Geometry: final body of the model. Coordinates: model frame, mm. A direction names the side the tool comes from. Give positions to 0.01 mm unless a question says otherwise; leave off trailing zeros. Write each loop counter-clockwise with the first axis right and the second up, starting at its lowest first coordinate (ties: lowest second). Pieces come first, ordered by that corner, then holes.
Q1. Pin query (flat end, axial travel): pin 1 (2 mm diameter, centred on x = -70.79, z = 29.92, fed in from +Y); pin 2 (12 mm diameter, centred on x = 68.5, y = -27, fed in from +Z); pin 3 (19 mm diameter, centred on x = -37.85, z = 12.07, fed in from +Y); pin 4 (2.5 mm diameter, centred on x = 21, y = 2, fed in from -Z). Return the tip coordinate at first contact, or that it passes through.
Q2. Reachability of faces 4 (the face through (-98.077, -11, 5)), 5 (the face through (-36.045, 1.014, 17.789)) from +Z, -Z, +X, -X, +Y, -Y: full face, straight path, thin tool, end or side. Return the list, or none.
Q3. Line query: L1, parallel to Z at x = -5, y = -8.5; L2, parallel to X at y = -10, z = -15; L3, parallel to X at y = -15, z = -20. Output: solid intervals per line, ascending.
Q4. Draft query along Z for faces 1 (the face through (-98.081, -0.105, 4.671)), 2 (the face through (58.796, 1.014, 18.266)), 3 (the face through (-1, -10, 68.577)). Return one class per face: pulls with the +Z half, pulls with the -Z half, needs draft (parallel to the pull), parting line crosses it, or undercut.
Q5. Cut plane C-C on x = -2. Return the cut outline in (y, z), plus the area to 3 significant figures.
Q6. Cut plane B-B on y = -26. Return the cut outline in (x, z).
Q7. Cut plane A-A on y = -11.5. Return the cut outline in (x, z).
```python
from build123d import *

# Parameters (mm, degrees)
SKETCH1_W           = 160
SKETCH1_H           = 117
BOSS_EXTRUDE1_DEPTH = 2
SKETCH3_R           = 6
CUT_EXTRUDE1_DEPTH  = 100.127443223
SKETCH4_R           = 6
CUT_EXTRUDE3_DEPTH  = 100.127443223
SKETCH5_R           = 6
CUT_EXTRUDE4_DEPTH  = 100.127443223
SKETCH6_W           = 76.000007526
SKETCH6_H           = 46.999987397
SKETCH6_W_2         = 72.000007526
SKETCH6_H_2         = 42.999987397
CUT_EXTRUDE5_DEPTH  = 10
SKETCH7_R           = 4
SKETCH7_R_2         = 1.25
BOSS_EXTRUDE2_DEPTH = 7.81
SKETCH8_W           = 78.000007526
SKETCH8_H           = 48.999987397
SKETCH8_W_2         = 76.000007526
SKETCH8_H_2         = 46.999987397
BOSS_EXTRUDE3_DEPTH = 5.19
SKETCH9_W           = 76.000007526
SKETCH9_H           = 46.999987397
BOSS_EXTRUDE4_DEPTH = 2
DRAFT2_ANGLE        = 35
SKETCH12_W          = 160
SKETCH12_H          = 14.938358446
SKETCH12_W_2        = 31.199462864
SKETCH12_H_2        = 9.099678356
SKETCH12_W_3        = 31.607152295
SKETCH12_H_3        = 7.36210802
CUT_EXTRUDE7_DEPTH  = 10
SKETCH13_R          = 6
CUT_EXTRUDE8_DEPTH  = 10
SKETCH14_W          = 120
SKETCH14_H          = 2
SKETCH14_W_2        = 2
SKETCH14_H_2        = 47
SKETCH14_H_3        = 27
SKETCH14_H_4        = 20
BOSS_EXTRUDE5_DEPTH = 8
SKETCH15_R          = 5
SKETCH15_R_2        = 4
BOSS_EXTRUDE6_DEPTH = 33.22
CHAMFER1_SIZE       = 5
SKETCH16_R          = 1.25
CUT_EXTRUDE9_DEPTH  = 10


with BuildPart() as part:
    # Sketch1 → Boss-Extrude1 (new body)
    with BuildSketch(Plane(origin=(0, 0, 0), x_dir=(1, 0, 0), z_dir=(0, 1, 0))):
        Rectangle(SKETCH1_W, SKETCH1_H)
    extrude(amount=BOSS_EXTRUDE1_DEPTH)

    # Sketch3 → Cut-Extrude1 (cut, through all)
    with BuildSketch(Plane(origin=(0, 2, 0), x_dir=(1, 0, 0), z_dir=(0, 1, 0))):
        with Locations(Location((72.15303621, -2.066282122, 0), (0, 0, 270))):
            Circle(SKETCH3_R)
    extrude(amount=-CUT_EXTRUDE1_DEPTH, mode=Mode.SUBTRACT)

    # Sketch4 → Cut-Extrude3 (cut, through all)
    with BuildSketch(Plane(origin=(0, 2, 0), x_dir=(1, 0, 0), z_dir=(0, 1, 0))):
        with Locations(Location((23.553035896, -50.866150132, 0), (0, 0, 270))):
            Circle(SKETCH4_R)
    extrude(amount=-CUT_EXTRUDE3_DEPTH, mode=Mode.SUBTRACT)

    # Sketch5 → Cut-Extrude4 (cut, through all)
    with BuildSketch(Plane(origin=(0, 2, 0), x_dir=(1, 0, 0), z_dir=(0, 1, 0))):
        with Locations(Location((64.653036213, -19.566282124, 0), (0, 0, 270))):
            Circle(SKETCH5_R)
        with Locations(Location((-37.846967603, -12.066282143, 0), (0, 0, 270))):
            Circle(SKETCH5_R)
        with Locations(Location((1.053035896, -50.866150137, 0), (0, 0, 270))):
            Circle(SKETCH5_R)
        with Locations(Location((-53.91492316, 3.900994062, 0), (0, 0, 270))):
            Circle(SKETCH5_R)
        with Locations(Location((-70.34696951, -12.066282149, 0), (0, 0, 270))):
            Circle(SKETCH5_R)
        with Locations(Location((-54.14683932, -28.466289977, 0), (0, 0, 270))):
            Circle(SKETCH5_R)
    extrude(amount=-CUT_EXTRUDE4_DEPTH, mode=Mode.SUBTRACT)

    # Sketch6 → Cut-Extrude5 (cut)
    with BuildSketch(Plane(origin=(0, 2, 0), x_dir=(1, 0, 0), z_dir=(0, 1, 0))):
        with Locations((11.764130909, -9.702217308)):
            Rectangle(SKETCH6_W, SKETCH6_H)
        with Locations((11.764130909, -9.702217308)):
            Rectangle(SKETCH6_W_2, SKETCH6_H_2, mode=Mode.SUBTRACT)
    extrude(amount=-CUT_EXTRUDE5_DEPTH, mode=Mode.SUBTRACT)


with BuildPart() as cut_extrude5_kept_piece:
    # of the separate pieces the step leaves, the one the design keeps (cut_extrude5_pieces_kept)
    add(part.part.solids().sort_by_distance((80, 0, 58.5))[0])

    # Sketch7 → Boss-Extrude2 (add)
    # profile 1 of 5: a face of its own
    with BuildSketch(Plane.XZ):
        with Locations(Location((66.701777656, -9.076203809, 0), (0, 0, 90))):
            Circle(SKETCH7_R)
        with Locations(Location((66.701777656, -9.076203809, 0), (0, 0, 270))):
            Circle(SKETCH7_R_2, mode=Mode.SUBTRACT)
    # profile 2 of 5: a face of its own
    with BuildSketch(Plane.XZ):
        with Locations(Location((63.702108967, 46.190679909, 0), (0, 0, 90))):
            Circle(SKETCH7_R)
        with Locations(Location((63.702108967, 46.190679909, 0), (0, 0, 270))):
            Circle(SKETCH7_R_2, mode=Mode.SUBTRACT)
    # profile 3 of 5: a face of its own
    with BuildSketch(Plane.XZ):
        with Locations(Location((-31.54560253, 48.927228564, 0), (0, 0, 90))):
            Circle(SKETCH7_R)
        with Locations(Location((-31.54560253, 48.927228564, 0), (0, 0, 270))):
            Circle(SKETCH7_R_2, mode=Mode.SUBTRACT)
    # profile 4 of 5: a face of its own
    with BuildSketch(Plane.XZ):
        with Locations(Location((-70.794006102, 29.915173129, 0), (0, 0, 90))):
            Circle(SKETCH7_R)
        with Locations(Location((-70.794006102, 29.915173129, 0), (0, 0, 270))):
            Circle(SKETCH7_R_2, mode=Mode.SUBTRACT)
    # profile 5 of 5: a face of its own
    with BuildSketch(Plane.XZ):
        with Locations(Location((-35.552994644, -4.584596423, 0), (0, 0, 90))):
            Circle(SKETCH7_R)
        with Locations(Location((-35.552994644, -4.584596423, 0), (0, 0, 270))):
            Circle(SKETCH7_R_2, mode=Mode.SUBTRACT)
    extrude(amount=BOSS_EXTRUDE2_DEPTH)

    # Sketch8 → Boss-Extrude3 (add)
    with BuildSketch(Plane(origin=(0, 2, 0), x_dir=(1, 0, 0), z_dir=(0, 1, 0))):
        with Locations((11.764130909, -9.702217308)):
            Rectangle(SKETCH8_W, SKETCH8_H)
        with Locations((11.764130909, -9.702217308)):
            Rectangle(SKETCH8_W_2, SKETCH8_H_2, mode=Mode.SUBTRACT)
    extrude(amount=BOSS_EXTRUDE3_DEPTH)

    # Sketch9 → Boss-Extrude4 (add)
    with BuildSketch(Plane(origin=(0, 7.19, 0), x_dir=(1, 0, 0), z_dir=(0, 1, 0))):
        with Locations((11.764130909, -9.702217308)):
            Rectangle(SKETCH9_W, SKETCH9_H)
        Polygon((-5.195084148, -31.43953726), (-6.695094805, -30.202211996), (-20.335872635, -30.202211996), (-20.335872635, 10.797777117), (43.864134191, 10.797777117), (43.864134191, -30.202211996), (30.223355703, -30.202211996), (28.723346116, -31.43953726), align=None, mode=Mode.SUBTRACT)
    extrude(amount=-BOSS_EXTRUDE4_DEPTH)

    # Draft2
    draft2_faces = [cut_extrude5_kept_piece.faces().sort_by_distance(p)[0] for p in [
        (11.764130909, 4.595, -14.79777639),
        (-27.235872854, 4.595, 9.702217309),
        (11.764130909, 4.595, 34.202211007),
        (50.764134672, 4.595, 9.702217309),
    ]]
    draft(draft2_faces, Plane.ZX.offset(7.19), DRAFT2_ANGLE)

    # Sketch12 → Cut-Extrude7 (cut)
    with BuildSketch(Plane(origin=(0, 2, 0), x_dir=(1, 0, 0), z_dir=(0, 1, 0))):
        with Locations((0, 51.030820777)):
            Rectangle(SKETCH12_W, SKETCH12_H)
        with Locations((-64.400268568, -53.950160822)):
            Rectangle(SKETCH12_W_2, SKETCH12_H_2)
        with Locations((64.196423853, -54.81894599)):
            Rectangle(SKETCH12_W_3, SKETCH12_H_3)
    extrude(amount=-CUT_EXTRUDE7_DEPTH, mode=Mode.SUBTRACT)

    # Sweep1: sweep along a path in Sketch10
    with BuildLine(Plane(origin=(0, 2, 0), x_dir=(1, 0, 0), z_dir=(0, 1, 0))) as sweep1_path:
        Line((-60, 58.5), (60, 58.5))
        ThreePointArc((60, 58.5), (88.284271247, 46.784271247), (100, 18.5))
        Line((100, 18.5), (100, -28.5))
        ThreePointArc((100, -28.5), (88.284271247, -56.784271247), (60, -68.5))
        Line((60, -68.5), (-60, -68.5))
        ThreePointArc((-60, -68.5), (-88.284271247, -56.784271247), (-100, -28.5))
        Line((-100, -28.5), (-100, 18.5))
        ThreePointArc((-100, 18.5), (-88.284271247, 46.784271247), (-60, 58.5))
    # Sketch11 → Sweep1 (sweep)
    with BuildSketch(Plane.XY.offset(8.5)):
        with BuildLine():
            Line((80, 2), (93.077362885, 2))
            ThreePointArc((93.077362885, 2), (98.027110354, -0.050252532), (100.077362885, -5))
            Line((100.077362885, -5), (100.077362885, -7.985538351))
            Line((100.077362885, -7.985538351), (98.077362885, -7.985538351))
            Line((98.077362885, -7.985538351), (98.077362885, -7))
            ThreePointArc((98.077362885, -7), (96.027110354, -2.050252532), (91.077362885, 0))
            Line((91.077362885, 0), (80, 0))
            Line((80, 0), (80, 2))
        make_face()
    sweep(path=sweep1_path.line)

    # Sketch13 → Cut-Extrude8 (cut)
    with BuildSketch(Plane(origin=(0, 2, 0), x_dir=(1, 0, 0), z_dir=(0, 1, 0))):
        with Locations(Location((1.053035896, -50.866150137, 0), (0, 0, 270))):
            Circle(SKETCH13_R)
        with Locations(Location((23.553035896, -50.866150132, 0), (0, 0, 270))):
            Circle(SKETCH13_R)
    extrude(amount=-CUT_EXTRUDE8_DEPTH, mode=Mode.SUBTRACT)

    # Sketch14 → Boss-Extrude5 (add)
    with BuildSketch(Plane.XZ.offset(7.985538351)):
        with Locations((0, 67.577362885)):
            Rectangle(SKETCH14_W, SKETCH14_H)
        with BuildLine():
            Line((-60, 66.577362885), (-60, 68.577362885))
            ThreePointArc((-60, 68.577362885), (-88.338975068, 56.838975068), (-100.077362885, 28.5))
            Line((-100.077362885, 28.5), (-98.077362885, 28.5))
            ThreePointArc((-98.077362885, 28.5), (-86.924761506, 55.424761506), (-60, 66.577362885))
        make_face()
        with Locations((-99.077362885, 5)):
            Rectangle(SKETCH14_W_2, SKETCH14_H_2)
        with BuildLine():
            ThreePointArc((-98.077362885, -18.5), (-86.924761506, -45.424761506), (-60, -56.577362885))
            Line((-60, -56.577362885), (-60, -58.577362885))
            ThreePointArc((-60, -58.577362885), (-88.338975068, -46.838975068), (-100.077362885, -18.5))
            Line((-100.077362885, -18.5), (-98.077362885, -18.5))
        make_face()
        with Locations((0, -57.577362885)):
            Rectangle(SKETCH14_W, SKETCH14_H)
        with BuildLine():
            ThreePointArc((60, -56.577362885), (86.924761506, -45.424761506), (98.077362885, -18.5))
            Line((98.077362885, -18.5), (100.077362885, -18.5))
            ThreePointArc((100.077362885, -18.5), (88.338975068, -46.838975068), (60, -58.577362885))
            Line((60, -58.577362885), (60, -56.577362885))
        make_face()
        with Locations((99.077362885, -5)):
            Rectangle(SKETCH14_W_2, SKETCH14_H_3)
        with Locations((99.077362885, 18.5)):
            Rectangle(SKETCH14_W_2, SKETCH14_H_4)
        with BuildLine():
            ThreePointArc((98.077362885, 28.5), (86.924761506, 55.424761506), (60, 66.577362885))
            Line((60, 66.577362885), (60, 68.577362885))
            ThreePointArc((60, 68.577362885), (88.338975068, 56.838975068), (100.077362885, 28.5))
            Line((100.077362885, 28.5), (98.077362885, 28.5))
        make_face()
    extrude(amount=BOSS_EXTRUDE5_DEPTH)

    # Sketch15 → Boss-Extrude6 (add)
    with BuildSketch(Plane.XZ):
        with Locations(Location((-50.604326003, -44.577362885, 0), (0, 0, 270))):
            Circle(SKETCH15_R)
        with Locations((87.077362885, -8.173505589)):
            Circle(SKETCH15_R_2)
    extrude(amount=BOSS_EXTRUDE6_DEPTH)

    # Chamfer1
    # the kernel refuses this chamfer: 5 mm, written as the material it adds along each edge
    with BuildSketch(Plane(origin=(-50.604326003, 0, -44.577362885), x_dir=(0, 0, -1), z_dir=(-1, 0, 0))) as chamfer1_piece_1:
        Polygon((5 + CHAMFER1_SIZE, 0), (5, CHAMFER1_SIZE), (5, 0), align=None)
    revolve(axis=Axis((-50.604326003, 0, -44.577362885), (0, -1, 0)))
    with BuildSketch(Plane(origin=(87.077362885, 0, -8.173505589), x_dir=(1, 0, 0), z_dir=(0, 0, -1))) as chamfer1_piece_2:
        Polygon((4 + CHAMFER1_SIZE, 0), (4, CHAMFER1_SIZE), (4, 0), align=None)
    revolve(axis=Axis((87.077362885, 0, -8.173505589), (0, -1, 0)))

    # Sketch16 → Cut-Extrude9 (cut)
    with BuildSketch(Plane.XZ.offset(33.22)):
        with Locations(Location((-50.604326003, -44.577362885, 0), (0, 0, 270))):
            Circle(SKETCH16_R)
        with Locations(Location((87.077362885, -8.173505589, 0), (0, 0, 270))):
            Circle(SKETCH16_R)
    extrude(amount=-CUT_EXTRUDE9_DEPTH, mode=Mode.SUBTRACT)


solid = cut_extrude5_kept_piece.part
```
Data:
1. pin 1: stops at y = 2
1. pin 2: passes through
1. pin 3: stops at y = 5.6
1. pin 4: stops at z = -55.57
2. face 4: -Y
2. face 5: +Y, -Y
3. L1: z = -58.58 to -56.58, 66.58 to 68.58
3. L2: x = -100.08 to -98.08, 98.08 to 100.08
3. L3: x = -100.05 to -98.05, 98.05 to 100.05
4. face 1: needs draft
4. face 2: undercut
4. face 3: pulls with the +Z half
5. outline: (-15.99, -58.58) - (-5, -58.58) arc R7 ccw to (2, -51.58) - (2, -18.43) - (7.19, -14.8) - (7.19, -10.8) - (5.19, -10.8) - (5.19, -13.8) - (0, -13.8) - (0, -49.58) arc R7 cw to (-7, -56.58) - (-15.99, -56.58) - close; (-15.99, 66.58) - (-7, 66.58) arc R7 cw to (0, 59.58) - (0, 56.03) - (2, 56.03) - (2, 61.58) arc R7 ccw to (-5, 68.58) - (-15.99, 68.58) - close; (0, 33.2) - (5.19, 33.2) - (5.19, 31.44) - (7.19, 31.44) - (7.19, 34.2) - (2, 37.84) - (2, 45.7) - (0, 45.7) - close
5. area: 242 mm2
6. outline: circle Ø10 at (-50.6, -44.58); circle Ø8 at (87.08, -8.17); hole circle Ø2.5 at (-50.6, -44.58); hole circle Ø2.5 at (87.08, -8.17)
7. outline: (-100.08, -18.5) arc R40.08 ccw to (-60, -58.58) - (60, -58.58) arc R40.08 ccw to (100.08, -18.5) - (100.08, 28.5) arc R40.08 ccw to (60, 68.58) - (-60, 68.58) arc R40.08 ccw to (-100.08, 28.5) - close; circle Ø10 at (-50.6, -44.58); circle Ø8 at (87.08, -8.17); hole (-98.08, -18.5) arc R38.08 ccw to (-60, -56.58) - (60, -56.58) arc R38.08 ccw to (98.08, -18.5) - (98.08, 28.5) arc R38.08 ccw to (60, 66.58) - (-60, 66.58) arc R38.08 ccw to (-98.08, 28.5) - close
